Verification items for this drawing (mm, ordinates from the low corner). A direction names the side the tool comes from. Coordinates: 2 decimals unless noted, no trailing zeros. Write each loop counter-clockwise with the first axis right and the second up, starting at its lowest first coordinate (ties: lowest second). Pieces come first, ordered by that corner, then holes. Notation, with made-up numbers: M -2,-16 L 43,-16 A30 cw 43,12 Z; hole C 54,89.25 d8. An arc over 180 degrees is marked long. Write each question's results on one line, items separated by ' | '.
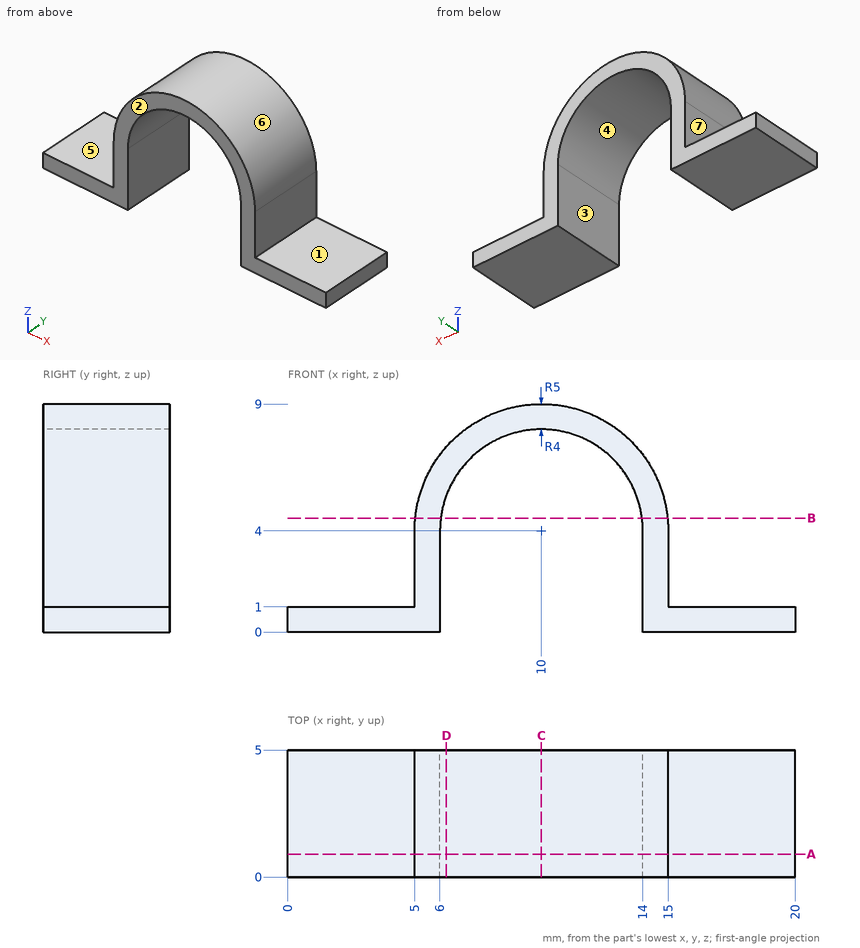
Q1. Sectioned sample at B-B on z = 4.5. Record the cut outline in (x, y).
Geometry check:
outline: M 5.03,0 L 6.03,0 L 6.03,5 L 5.03,5 Z; M 13.97,0 L 14.97,0 L 14.97,5 L 13.97,5 Z
Q2. Access from +Z, -Z, +X, -X, +Y, -Y to the whole of each face (thin tool, end or side, straight path). Record for the marked faces 1, 2 and 3.
Geometry check:
face 1: +Z, +X, +Y, -Y | face 2: +Z, -Z, +X, -X, -Y | face 3: -Z, +Y, -Y
Q3. Sectioned sample at A-A on y = 0.9. Record the cut outline in (x, z), and give its area (3 significant figures).
Geometry check:
outline: M 0,0 L 6,0 L 6,4 A4 cw 14,4 L 14,0 L 20,0 L 20,1 L 15,1 L 15,4 A5 ccw 5,4 L 5,1 L 0,1 Z | area: 32.1 mm2
Q4. Scan lines: probe 1 along X at (y, z) = (3.8, 2.25); probe 2 along Z at (x, y) = (16.25, 3.75); probe 3 along X at (y, z) = (4.15, 6). Record each from-to range of solid material in increasing order.
Geometry check:
probe 1: x = 5 to 6, 14 to 15 | probe 2: z = 0 to 1 | probe 3: x = 5.42 to 6.54, 13.46 to 14.58
Q5. Sectioned sample at D-D on x = 6.25. Record the cut outline in (y, z).
Geometry check:
outline: M 0,5.39 L 5,5.39 L 5,7.31 L 0,7.31 Z
Q6. Sectioned sample at C-C on x = 10. Record the cut outline in (y, z), and give its area (3 significant figures).
Geometry check:
outline: M 0,8 L 5,8 L 5,9 L 0,9 Z | area: 5.00 mm2
Q7. Mould release check, pull along X, two halves, no side actions. Record for the marked faces 4, 5, 6 and 7: pulls with the +X half, pulls with the -X half, needs draft (parallel to the pull), parting line crosses it, or undercut.
Geometry check:
face 4: undercut | face 5: needs draft | face 6: parting line crosses it | face 7: pulls with the -X half
Q8. Depth check by flat-ended pin: P1, Ø2, axis at y = 4, z = 7, coming from the +X side; P2, Ø0.9, axis at y = 3.5, z = 3, coming from the +X side; P3, Ø3, axis at y = 3.5, z = 3, coming from the -X side. Enter the tip coordinate at first touch or a pass-through.
Geometry check:
P1: stops at x = 14.58 | P2: stops at x = 15 | P3: stops at x = 5
